Job drawing, mm, ordinate dimensions from the low corner. One solid piece. Round coordinates to 2 decimals unless told otherwise and drop trailing zeros. Order: outer loops, then holes, each group sorted by start corner. A loop starts at its lowest first (then second) coordinate and runs counter-clockwise, first axis right, second up. Notation, with made-up numbers: (-27.75, 43.25) -> (5.25, 43.25) arc R23 cw to (5.25, 80.25) -> close; hole circle Ø11 at (83.25, 66.5). An arc over 180 degrees is marked (long way). Answer as a JSON object with one key per item and string values. Group by question number.
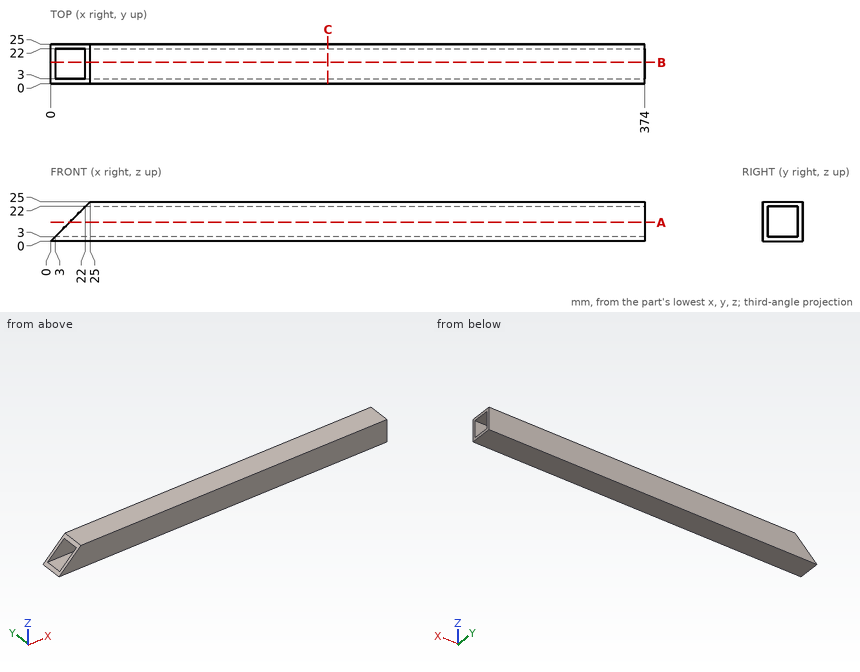
Q1. Wall check: line 1 (Z direction, x = 226.5, y = 14); line 2 (X direction, y = 22.25, z = 17.5). Give the ranges that are in metal, low to high. Write a range as [from, to].
Q2. Drop a flat-ended pin along its axis: pin 1 Ø12 at (x, z) = (124, 18) entering from -Y. Give the stop position or say it passes through.
Q3. Band-saw the part on B-B (y = 13.5). List the corners of the cut face in (x, z), plus the area to 3 significant figures.
Q4. Band-saw the part on C-C (x = 174.5). List the corners of the cut face in (y, z), plus the area to 3 significant figures.
Q5. Band-saw the part on A-A (z = 12). List the corners of the cut face in (x, y), plus the area to 3 significant figures.
Completed:
{
 "1": {"line 1": "[0, 3], [22, 25]", "line 2": "[17.5, 374]"},
 "2": {"pin 1": "y = 0"},
 "3": {"outline": "(0, 0) -> (374, 0) -> (374, 3) -> (3, 3) -> close; (22, 22) -> (374, 22) -> (374, 25) -> (25, 25) -> close", "area": "2,170 mm2"},
 "4": {"outline": "(0, 0) -> (25, 0) -> (25, 25) -> (0, 25) -> close; hole (3, 3) -> (22, 3) -> (22, 22) -> (3, 22) -> close", "area": "264 mm2"},
 "5": {"outline": "(12, 0) -> (374, 0) -> (374, 3) -> (12, 3) -> close; (12, 22) -> (374, 22) -> (374, 25) -> (12, 25) -> close", "area": "2,170 mm2"}
}
